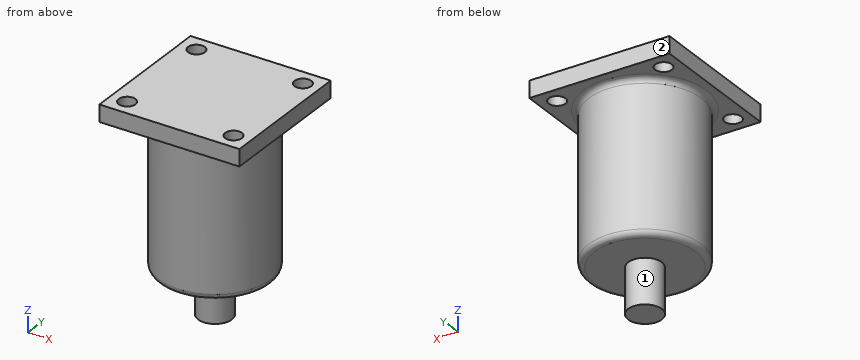
from build123d import *

# Parameters (mm, degrees)
SKETCH_2_W          = 25
SKETCH_2_H          = 25
EXTRUDE_1_DEPTH     = 3
SKETCH_3_R          = 1.5
CUT_EXTRUDE_2_DEPTH = 4
EXTRUDE_START       = -3
SKETCH_4_R          = 10
EXTRUDE_2_DEPTH     = 27
SKETCH_5_R          = 3
EXTRUDE_3_DEPTH     = 8
FILLET_3_R          = 1


with BuildPart() as part:
    # 草图2 → 凸台-拉伸1 (new body)
    with BuildSketch(Plane.XY):
        with Locations((12.5, -12.5)):
            Rectangle(SKETCH_2_W, SKETCH_2_H)
    extrude(amount=EXTRUDE_1_DEPTH)

    # 草图3 → 切除-拉伸2 (cut, through all)
    with BuildSketch(Plane(origin=(0, 0, 0), x_dir=(-1, 0, 0), z_dir=(0, 0, -1))):
        with Locations((-22, -3)):
            Circle(SKETCH_3_R)
        with Locations((-3, -3)):
            Circle(SKETCH_3_R)
        with Locations((-3, -22)):
            Circle(SKETCH_3_R)
        with Locations((-22, -22)):
            Circle(SKETCH_3_R)
    extrude(amount=-CUT_EXTRUDE_2_DEPTH, mode=Mode.SUBTRACT)

    # 草图4 → 凸台-拉伸2 (add)
    with BuildSketch(Plane.XY.offset(3).offset(EXTRUDE_START)):
        with Locations((12.5, -12.5)):
            Circle(SKETCH_4_R)
    extrude(amount=-EXTRUDE_2_DEPTH)

    # 草图5 → 凸台-拉伸3 (add)
    with BuildSketch(Plane(origin=(0, 0, -27), x_dir=(-1, 0, 0), z_dir=(0, 0, -1))):
        with Locations((-12.5, -12.5)):
            Circle(SKETCH_5_R)
    extrude(amount=EXTRUDE_3_DEPTH)

    # 圆角3
    fillet_3_edges = [part.edges().sort_by_distance(p)[0] for p in [
        (2.5, -12.5, -27),
        (2.5, -12.5, 0),
    ]]
    fillet(fillet_3_edges, radius=FILLET_3_R)


solid = part.part
Could you check a few things on this model? Use its own coordinates, in mm. Face numbers are marked on the shaded views. A direction names the side the tool comes from. Give positions to 0.01 mm unless a question says otherwise; leave off trailing zeros. Order: outer loops, then holes, each group sorted by start corner. A loop starts at its lowest first (then second) coordinate and runs counter-clockwise, first axis right, second up. Notation, with made-up numbers: (57, 36) - (88, 36) arc R8 ccw to (88, 47) - close; hole circle Ø11 at (-35, 84). An arc over 180 degrees is marked (long way). Return JSON: item names as keys, results as strings. Group by question number.
Q1. Suppose I cut it at D-D, the plane y = -22. State how many separate pieces and enclosed holes the cut face has, and give its area (3 significant figures).
Q2. Suppose I cut it at B-B, the plane y = -12.5. Please give me the cut outline in (x, z), and give its area (3 significant figures).
Q3. Suppose I cut it at C-C, the plane z = -15.5. Please give me the cut outline in (x, y), and give its area (3 significant figures).
Q4. Please list where these lines run through material, in increasing order: line 1 along Y through (x, z) = (22, 2.2); line 2 along Z through (x, y) = (9.5, -19); line 3 along Z through (x, y) = (1.75, -19.25). Write a range as [from, to].
Q5. Suppose I cut it at A-A, the plane x = 12.5. Please give me the cut outline in (y, z).
Q6. Will these pins go through, and if not, where does the flat tip stop? pin 1 Ø1 at (x, z) = (16, -16.5) entering from -Y; pin 2 Ø2 at (y, z) = (-5.5, -2.5) entering from -X; pin 3 Ø2 at (y, z) = (-11, -12) entering from +X; pin 4 Ø2.5 at (x, y) = (22, -22) entering from -Z.
Q7. Which directions (+Z, -Z, +X, -X, +Y, -Y) give clear straight access to the entire face, cutting with the end or side of a thin tool? Please do the marked faces 1 and 2.
Resolved:
{
 "1": {"separate pieces": "3", "enclosed holes": "0", "area": "225 mm2"},
 "2": {"outline": "(0, 0) - (1.5, 0) arc R1 cw to (2.5, -1) - (2.5, -26) arc R1 ccw to (3.5, -27) - (9.5, -27) - (9.5, -35) - (15.5, -35) - (15.5, -27) - (21.5, -27) arc R1 ccw to (22.5, -26) - (22.5, -1) arc R1 cw to (23.5, 0) - (25, 0) - (25, 3) - (0, 3) - close", "area": "663 mm2"},
 "3": {"outline": "circle Ø20 at (12.5, -12.5)", "area": "314 mm2"},
 "4": {"line 1": "y = [-25, -23.5], [-20.5, -4.5], [-1.5, 0]", "line 2": "z = [-27, 3]", "line 3": "z = [0, 3]"},
 "5": {"outline": "(-25, 0) - (-23.5, 0) arc R1 cw to (-22.5, -1) - (-22.5, -26) arc R1 ccw to (-21.5, -27) - (-15.5, -27) - (-15.5, -35) - (-9.5, -35) - (-9.5, -27) - (-3.5, -27) arc R1 ccw to (-2.5, -26) - (-2.5, -1) arc R1 cw to (-1.5, 0) - (0, 0) - (0, 3) - (-25, 3) - close"},
 "6": {"pin 1": "stops at y = -22.04", "pin 2": "stops at x = 4.5", "pin 3": "stops at x = 22.49", "pin 4": "passes through"},
 "7": {"face 1": "-Z", "face 2": "+Z, -Z, +X, -X, +Y"}
}
